from build123d import *

# Parameters (mm, degrees)
SKETCH1_W           = 12.7
SKETCH1_H           = 12.7
SKETCH1_W_2         = 9.4
SKETCH1_H_2         = 9.4
BOSS_EXTRUDE1_DEPTH = 175
CUT_EXTRUDE1_DEPTH  = 13.7


with BuildPart() as part:
    # Sketch1 → Boss-Extrude1 (new body)
    with BuildSketch(Plane.XY):
        Rectangle(SKETCH1_W, SKETCH1_H)
        Rectangle(SKETCH1_W_2, SKETCH1_H_2, mode=Mode.SUBTRACT)
    extrude(amount=BOSS_EXTRUDE1_DEPTH)

    # Sketch2 → Cut-Extrude1 (cut, through all)
    with BuildSketch(Plane(origin=(0, 6.35, 0), x_dir=(1, 0, 0), z_dir=(0, 1, 0))):
        with BuildLine():
            Line((-6.35, -3.175), (-6.35, 0))
            Line((-6.35, 0), (-3.175, 0))
            ThreePointArc((-3.175, 0), (-5.42006403, -0.92993597), (-6.35, -3.175))
        make_face()
        with BuildLine():
            Line((3.175, 0), (6.35, 0))
            Line((6.35, 0), (6.35, -3.175))
            ThreePointArc((6.35, -3.175), (5.42006403, -0.92993597), (3.175, 0))
        make_face()
    extrude(amount=-CUT_EXTRUDE1_DEPTH, mode=Mode.SUBTRACT)


solid = part.part
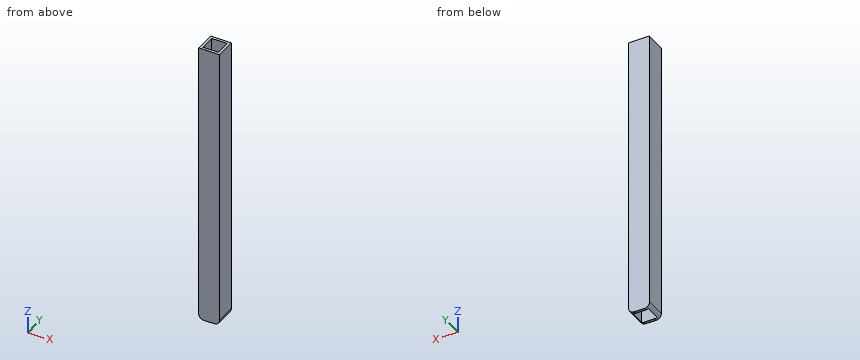
Can you work these out from the model? Positions are in its coordinate system, mm. Round coordinates to 2 decimals unless told otherwise and drop trailing zeros. Order: outer loops, then holes, each group sorted by start corner. A loop starts at its lowest first (then second) coordinate and runs counter-clockwise, first axis right, second up. Notation, with made-up numbers: (-7.5, 62.5) - (3.5, 62.5) arc R15 cw to (3.5, 76.5) - close; hole circle Ø9 at (72.25, 33.5). An arc over 180 degrees is marked (long way). Answer in a Markdown table with one row per item.
(1) Suppose I cut it at C-C, the plane z = 79. Please give me the cut outline in (x, y).
From the geometry:
| item | result |
|---|---|
| outline | (-6.35, -6.35) - (6.35, -6.35) - (6.35, 6.35) - (-6.35, 6.35) - close; hole (-4.7, -4.7) - (4.7, -4.7) - (4.7, 4.7) - (-4.7, 4.7) - close |
(2) Suppose I cut it at B-B, the plane y = -1. Please give me the cut outline in (x, z) (3 decimals), plus the area to 3 significant figures.
From the geometry:
| item | result |
|---|---|
| outline | (-6.35, 3.175) arc R3.175 ccw to (-4.7, 0.39) - (-4.7, 175) - (-6.35, 175) - close; (4.7, 0.39) arc R3.175 ccw to (6.35, 3.175) - (6.35, 175) - (4.7, 175) - close |
| area | 574 mm2 |
(3) Please list where these lines run through material, in increasing order: L1, parallel to X at y = -0.5, z = 38.5; L2, parallel to Z at x = 4.75, y = -5. Write a range as from..to.
From the geometry:
| item | result |
|---|---|
| L1 | x = -6.35..-4.7, 4.7..6.35 |
| L2 | z = 0.42..175 |
(4) Suppose I cut it at A-A, the plane x = 1.75. Please give me the cut outline in (y, z).
From the geometry:
| item | result |
|---|---|
| outline | (-6.35, 0) - (-4.7, 0) - (-4.7, 175) - (-6.35, 175) - close; (4.7, 0) - (6.35, 0) - (6.35, 175) - (4.7, 175) - close |
(5) For P1, Ø1.5, axis at x = 3, y = -3, coming from the -Z side, with a flat end and sliding along its axis, tell me the tip position at first contact or that it passes through.
From the geometry:
| item | result |
|---|---|
| P1 | passes through |
